```python
from build123d import *

# Parameters (mm, degrees)
SKETCH1_R           = 8
BOSS_EXTRUDE1_DEPTH = 10
SKETCH2_R           = 5
BOSS_EXTRUDE2_DEPTH = 70
CHAMFER1_SIZE       = 1


with BuildPart() as part:
    # Sketch1 → Boss-Extrude1 (new body)
    with BuildSketch(Plane(origin=(0, 0, 0), x_dir=(1, 0, 0), z_dir=(0, 1, 0))):
        Circle(SKETCH1_R)
    extrude(amount=BOSS_EXTRUDE1_DEPTH)

    # Sketch2 → Boss-Extrude2 (add)
    with BuildSketch(Plane.XZ):
        Circle(SKETCH2_R)
    extrude(amount=BOSS_EXTRUDE2_DEPTH)

    # Chamfer1
    chamfer1_edges = [part.edges().sort_by_distance(p)[0] for p in [
        (-5, -70, 0),
    ]]
    chamfer(chamfer1_edges, length=CHAMFER1_SIZE)


solid = part.part
```
Work out the finished part from the listing and answer in its coordinate system (mm). A direction names the side the tool comes from. Coordinates: 2 decimals unless noted, no trailing zeros. Loops run counter-clockwise (first coordinate to the right, second up) from the corner with the lowest first, then second, coordinate; pieces in that order, holes last. Notation, with made-up numbers: (54.25, -1.5) - (82.25, -1.5) arc R11 ccw to (82.25, 8.5) - close; hole circle Ø1 at (10.5, -14.5). An arc over 180 degrees is marked (long way). Use a Markdown table: item, result.
Item 1: Consider probe 1 along Y at (x, z) = (2.5, -6.25); probe 2 along X at (y, z) = (-20, -4.25); probe 3 along X at (y, z) = (1, 4). Determine where each line is inside the solid, lowest interval first. Write a range as from..to.
Evaluation:
| item | result |
|---|---|
| probe 1 | y = 0..10 |
| probe 2 | x = -2.63..2.63 |
| probe 3 | x = -6.93..6.93 |
Item 2: Find section C-C, the plane y = -57. Determine the outline of the cut face in (x, z), and give its area (3 significant figures).
Evaluation:
| item | result |
|---|---|
| outline | circle Ø10 at (0, 0) |
| area | 78.5 mm2 |
Item 3: Find section A-A, the plane x = 0. Determine the outline of the cut face in (y, z), and give its area (3 significant figures).
Evaluation:
| item | result |
|---|---|
| outline | (-70, -4) - (-69, -5) - (0, -5) - (0, -8) - (10, -8) - (10, 8) - (0, 8) - (0, 5) - (-69, 5) - (-70, 4) - close |
| area | 859 mm2 |
Item 4: Find section B-B, the plane z = 0. Determine the outline of the cut face in (x, y), and give its area (3 significant figures).
Evaluation:
| item | result |
|---|---|
| outline | (-8, 0) - (-5, 0) - (-5, -69) - (-4, -70) - (4, -70) - (5, -69) - (5, 0) - (8, 0) - (8, 10) - (-8, 10) - close |
| area | 859 mm2 |
Item 5: For faces 1 (the cylindrical face through (-1.08, -34.02, -4.88)), 2 (the cylindrical face through (-1.73, 4.93, 7.81)), determine the directions among +Z, -Z, +X, -X, +Y, -Y from which every point of the face is accessible in a straight line to the end or side of a thin tool.
Evaluation:
| item | result |
|---|---|
| face 1 | -Y |
| face 2 | +Y, -Y |
Item 6: Given pin 1 Ø3 at (x, z) = (4.5, 6) entering from -Y; pin 2 Ø2 at (y, z) = (-42.5, 5) entering from +X; pin 3 Ø4 at (x, y) = (-5.5, -60) entering from -Z, each flat-ended and moving along its own axis, determine where each tip first touches the part or whether it passes through.
Evaluation:
| item | result |
|---|---|
| pin 1 | stops at y = 0 |
| pin 2 | stops at x = 3 |
| pin 3 | stops at z = -3.57 |
